Verification items for this drawing (mm, ordinates from the low corner). A direction names the side the tool comes from. Round coordinates to 2 decimals unless told otherwise and drop trailing zeros. Write each loop counter-clockwise with the first axis right and the second up, starting at its lowest first coordinate (ties: lowest second). Pieces come first, ordered by that corner, then holes. Notation, with made-up numbers: (8, 37) -> (64, 37) arc R28 ccw to (64, 62) -> close; hole circle Ø11 at (-25.75, 71). An arc over 180 degrees is marked (long way). One line per item, written item: value.
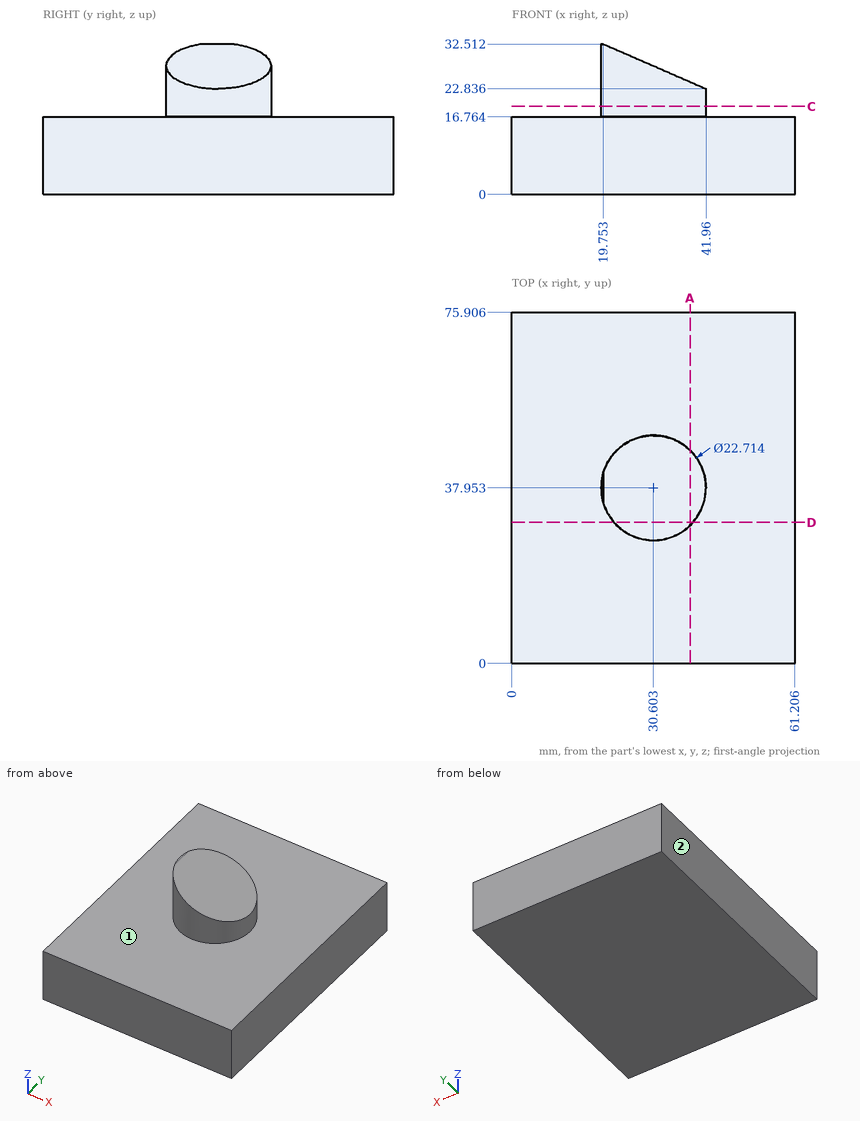
Item 1: Sectioned sample at C-C (z = 19). Enter the section's corners in (x, y).
Result set:
outline: circle Ø22.71 at (30.6, 37.95)
Item 2: Tool access check on the marked faces 1 and 2. Record the directions out of +Z, -Z, +X, -X, +Y, -Y that give a thin tool (end or side, any length) a straight path to the whole face; none if there is none.
Result set:
face 1: +Z
face 2: +Z, -Z, -X, +Y, -Y
Item 3: Sectioned sample at A-A (x = 38.5). Enter the section's corners in (y, z) (1 decimal).
Result set:
outline: (0, 0) -> (75.9, 0) -> (75.9, 16.8) -> (46.1, 16.8) -> (46.1, 24.3) -> (29.8, 24.3) -> (29.8, 16.8) -> (0, 16.8) -> close
Item 4: Material ranges on line 1 along Y through (x, z) = (30, 24.5); line 2 along Z through (x, y) = (51.5, 39); line 3 along Y through (x, z) = (33, 25.5) (1 decimal), recorded low to high.
Result set:
line 1: 26.61 to 49.29
line 2: 0 to 16.76
line 3: 26.9 to 49.1
Item 5: Depth check by flat-ended pin: pin 1 (3 mm diameter, centred on y = 35.5, z = 25, fed in from -X); pin 2 (5 mm diameter, centred on x = 22, z = 22.5, fed in from +Y); pin 3 (2 mm diameter, centred on x = 28, y = 21, fed in from +Z); pin 4 (1 mm diameter, centred on x = 18, z = 28.5, fed in from -Y). Enter the tip coordinate at first touch or a pass-through.
Result set:
pin 1: x = 19.29
pin 2: y = 47.53
pin 3: z = 16.76
pin 4: through
Item 6: Sectioned sample at D-D (y = 30.5). Enter the section's corners in (x, z).
Result set:
outline: (0, 0) -> (61.21, 0) -> (61.21, 16.76) -> (39.17, 16.76) -> (39.17, 24.05) -> (22.03, 31.52) -> (22.03, 16.76) -> (0, 16.76) -> close
